from build123d import *

# Parameters (mm, degrees)
SKETCH1_W           = 25.4
SKETCH1_H           = 50.8
BOSS_EXTRUDE1_DEPTH = 2.00000108
SKETCH2_W           = 25.4
SKETCH2_H           = 50.8
SKETCH2_W_2         = 23.39999892
SKETCH2_H_2         = 48.79999892
BOSS_EXTRUDE2_DEPTH = 4.999999906
FILLET1_R           = 2.000000064
FILLET2_R           = 1.000000032
CUT_EXTRUDE3_REACH  = 52.8
SKETCH6_R           = 2.2225
CUT_EXTRUDE4_REACH  = 52.8
SKETCH7_W           = 7.62
SKETCH7_H           = 3.81
CUT_EXTRUDE5_REACH  = 27.4
SKETCH8_W           = 2.54
SKETCH8_H           = 2.54
CUT_EXTRUDE6_REACH  = 9
SKETCH9_R           = 1.27


with BuildPart() as part:
    # Sketch1 → Boss-Extrude1 (new body)
    with BuildSketch(Plane.XY):
        with Locations((12.7, 25.4)):
            Rectangle(SKETCH1_W, SKETCH1_H)
    extrude(amount=BOSS_EXTRUDE1_DEPTH)

    # Sketch2 → Boss-Extrude2 (add)
    with BuildSketch(Plane.XY.offset(2.00000108)):
        with Locations((12.7, 25.4)):
            Rectangle(SKETCH2_W, SKETCH2_H)
        with Locations((12.7, 25.4)):
            Rectangle(SKETCH2_W_2, SKETCH2_H_2, mode=Mode.SUBTRACT)
    extrude(amount=BOSS_EXTRUDE2_DEPTH)

    # Fillet1
    fillet1_edges = [part.edges().sort_by_distance(p)[0] for p in [
        (0, 50.8, 3.500000493),
        (25.4, 50.8, 3.500000493),
        (25.4, 0, 3.500000493),
        (0, 0, 3.500000493),
    ]]
    fillet(fillet1_edges, radius=FILLET1_R)

    # Fillet2
    fillet2_edges = [part.edges().sort_by_distance(p)[0] for p in [
        (12.7, 0, 0),
        (0, 25.4, 0),
        (12.7, 50.8, 0),
        (25.4, 25.4, 0),
        (24.814213544, 50.214213544, 0),
        (0.585786456, 50.214213544, 0),
        (24.814213544, 0.585786456, 0),
        (0.585786456, 0.585786456, 0),
    ]]
    fillet(fillet2_edges, radius=FILLET2_R)

    # Sketch6 → Cut-Extrude3 (cut, up to next)
    with BuildSketch(Plane(origin=(0, 50.8, 0), x_dir=(1, 0, 0), z_dir=(0, 1, 0)), mode=Mode.PRIVATE) as cut_extrude3_sk1:
        with Locations((18.319999936, -4.460000986)):
            Circle(SKETCH6_R)
    cut_extrude3_tool1 = extrude(cut_extrude3_sk1.sketch, amount=-CUT_EXTRUDE3_REACH, mode=Mode.PRIVATE) & part.part
    add(cut_extrude3_tool1.solids().sort_by_distance((18.32, 50.8, 4.460001))[0], mode=Mode.SUBTRACT)

    # Sketch7 → Cut-Extrude4 (cut, up to next)
    with BuildSketch(Plane(origin=(0, 50.8, 0), x_dir=(1, 0, 0), z_dir=(0, 1, 0)), mode=Mode.PRIVATE) as cut_extrude4_sk1:
        with Locations((10.699999936, -5.095000986)):
            Rectangle(SKETCH7_W, SKETCH7_H)
    cut_extrude4_tool1 = extrude(cut_extrude4_sk1.sketch, amount=-CUT_EXTRUDE4_REACH, mode=Mode.PRIVATE) & part.part
    add(cut_extrude4_tool1.solids().sort_by_distance((10.7, 50.8, 5.095001))[0], mode=Mode.SUBTRACT)

    # Sketch8 → Cut-Extrude5 (cut, up to next)
    with BuildSketch(Plane.ZY, mode=Mode.PRIVATE) as cut_extrude5_sk1:
        with Locations((5.730000986, 39.909999936)):
            Rectangle(SKETCH8_W, SKETCH8_H)
    cut_extrude5_tool1 = extrude(cut_extrude5_sk1.sketch, amount=-CUT_EXTRUDE5_REACH, mode=Mode.PRIVATE) & part.part
    add(cut_extrude5_tool1.solids().sort_by_distance((0, 39.91, 5.730001))[0], mode=Mode.SUBTRACT)
    # Sketch8 → Cut-Extrude5 (cut, up to next)
    with BuildSketch(Plane.ZY, mode=Mode.PRIVATE) as cut_extrude5_sk2:
        with Locations((5.730000986, 29.749999936)):
            Rectangle(SKETCH8_W, SKETCH8_H)
    cut_extrude5_tool2 = extrude(cut_extrude5_sk2.sketch, amount=-CUT_EXTRUDE5_REACH, mode=Mode.PRIVATE) & part.part
    add(cut_extrude5_tool2.solids().sort_by_distance((0, 29.75, 5.730001))[0], mode=Mode.SUBTRACT)

    # Sketch9 → Cut-Extrude6 (cut, up to next)
    with BuildSketch(Plane(origin=(0, 0, 0), x_dir=(-1, 0, 0), z_dir=(0, 0, -1)), mode=Mode.PRIVATE) as cut_extrude6_sk1:
        with Locations((-3.540000032, 9.890000032)):
            Circle(SKETCH9_R)
    cut_extrude6_tool1 = extrude(cut_extrude6_sk1.sketch, amount=-CUT_EXTRUDE6_REACH, mode=Mode.PRIVATE) & part.part
    add(cut_extrude6_tool1.solids().sort_by_distance((3.54, 9.89, 0))[0], mode=Mode.SUBTRACT)
    # Sketch9 → Cut-Extrude6 (cut, up to next)
    with BuildSketch(Plane(origin=(0, 0, 0), x_dir=(-1, 0, 0), z_dir=(0, 0, -1)), mode=Mode.PRIVATE) as cut_extrude6_sk2:
        with Locations((-3.540000032, 13.700000032)):
            Circle(SKETCH9_R)
    cut_extrude6_tool2 = extrude(cut_extrude6_sk2.sketch, amount=-CUT_EXTRUDE6_REACH, mode=Mode.PRIVATE) & part.part
    add(cut_extrude6_tool2.solids().sort_by_distance((3.54, 13.7, 0))[0], mode=Mode.SUBTRACT)
    # Sketch9 → Cut-Extrude6 (cut, up to next)
    with BuildSketch(Plane(origin=(0, 0, 0), x_dir=(-1, 0, 0), z_dir=(0, 0, -1)), mode=Mode.PRIVATE) as cut_extrude6_sk3:
        with Locations((-3.540000032, 17.510000032)):
            Circle(SKETCH9_R)
    cut_extrude6_tool3 = extrude(cut_extrude6_sk3.sketch, amount=-CUT_EXTRUDE6_REACH, mode=Mode.PRIVATE) & part.part
    add(cut_extrude6_tool3.solids().sort_by_distance((3.54, 17.51, 0))[0], mode=Mode.SUBTRACT)


solid = part.part
Geometry check sheet. Reference: the model listing, model coordinates, mm. A direction names the side the tool comes from. Give positions to 0.01 mm unless a question says otherwise; leave off trailing zeros. Write each loop counter-clockwise with the first axis right and the second up, starting at its lowest first coordinate (ties: lowest second). Pieces come first, ordered by that corner, then holes. Notation, with made-up numbers: M 10,52 L 47,52 A29 ccw 47,86 Z; hole C 18,45.5 d2. An arc over 180 degrees is marked long. One line per question, with ' | ' between items.
1. Gauge pin test, flat ends, axial feed: pin 1 (4 mm diameter, centred on x = 3.54, y = 13.7, fed in from -Z); pin 2 (0.5 mm diameter, centred on x = 0.5, y = 39.5, fed in from +Z); pin 3 (1.5 mm diameter, centred on x = 4, y = 21, fed in from +Z); pin 4 (1.1 mm diameter, centred on x = 0.5, z = 6, fed in from -Y). Record the tip position at first contact, or that the pin passes through.
Ans:
pin 1: z = 0 | pin 2: z = 4.46 | pin 3: z = 2 | pin 4: y = 0.24
2. Scan lines: line 1 along Y through (x, z) = (3.54, 1.25); line 2 along Y through (x, z) = (22, 4.25); line 3 along X through (y, z) = (3.5, 5.75). Record each from-to range of solid material in increasing order. Write a range as from..to.
Ans:
line 1: 0..8.62, 11.16..12.43, 14.97..16.24, 18.78..50.8 | line 2: 0..1, 49.8..50.8 | line 3: 0..1, 24.4..25.4
3. Cross-section at C-C (z = 5). Enter the section's corners in (x, y).
Ans:
outline: M 0,2 A2 ccw 2,0 L 23.4,0 A2 ccw 25.4,2 L 25.4,48.8 A2 ccw 23.4,50.8 L 20.48,50.8 L 20.48,49.8 L 24.4,49.8 L 24.4,1 L 1,1 L 1,28.48 L 0,28.48 Z; M 0,31.02 L 1,31.02 L 1,38.64 L 0,38.64 Z; M 0,41.18 L 1,41.18 L 1,49.8 L 6.89,49.8 L 6.89,50.8 L 2,50.8 A2 ccw 0,48.8 Z; M 14.51,49.8 L 16.16,49.8 L 16.16,50.8 L 14.51,50.8 Z
4. Cross-section at B-B (y = 9.89). Enter the section's corners in (x, z).
Ans:
outline: M 0,1 A1 ccw 1,0 L 2.27,0 L 2.27,2 L 1,2 L 1,7 L 0,7 Z; M 4.81,0 L 24.4,0 A1 ccw 25.4,1 L 25.4,7 L 24.4,7 L 24.4,2 L 4.81,2 Z
5. Cross-section at D-D (x = 16.75). Enter the section's corners in (y, z), plus the area to 3 significant figures.
Ans:
outline: M 0,1 A1 ccw 1,0 L 49.8,0 A1 ccw 50.8,1 L 50.8,2.89 L 49.8,2.89 L 49.8,2 L 1,2 L 1,7 L 0,7 Z; M 49.8,6.03 L 50.8,6.03 L 50.8,7 L 49.8,7 Z | area: 108 mm2
6. Cross-section at A-A (x = 3.54). Enter the section's corners in (y, z).
Ans:
outline: M 0,1 A1 ccw 1,0 L 8.62,0 L 8.62,2 L 1,2 L 1,7 L 0,7 Z; M 11.16,0 L 12.43,0 L 12.43,2 L 11.16,2 Z; M 14.97,0 L 16.24,0 L 16.24,2 L 14.97,2 Z; M 18.78,0 L 49.8,0 A1 ccw 50.8,1 L 50.8,7 L 49.8,7 L 49.8,2 L 18.78,2 Z
7. Set-up check for faces 4 (the face through (0.57, 0.6, 4.04)), 5 (the face through (13, 49.8, 3)), 6 (the face through (0.5, 29.7, 4.46)), 7 (the face through (25.4, 25, 4)), 8 (the face through (14.51, 50, 5)): record each of +Z, -Z, +X, -X, +Y, -Y from which the full face is reachable in a straight line by a thin tool's end or side.
Ans:
face 4: +Z, -Z, -X, -Y | face 5: +Z | face 6: +Z, -X | face 7: +Z, -Z, +X, +Y, -Y | face 8: +Z, +Y
8. Mould release check, pull along Y, two halves, no side actions. Record for faces 1 (the face through (0.5, 34.9, 7)), 2 (the face through (2.954, 8.763, 0.986)), 3 (the face through (0.57, 50.2, 3.96)): released by +Y, released by -Y, zero draft, split by the parting line, or undercut.
Ans:
face 1: zero draft | face 2: undercut | face 3: released by +Y
